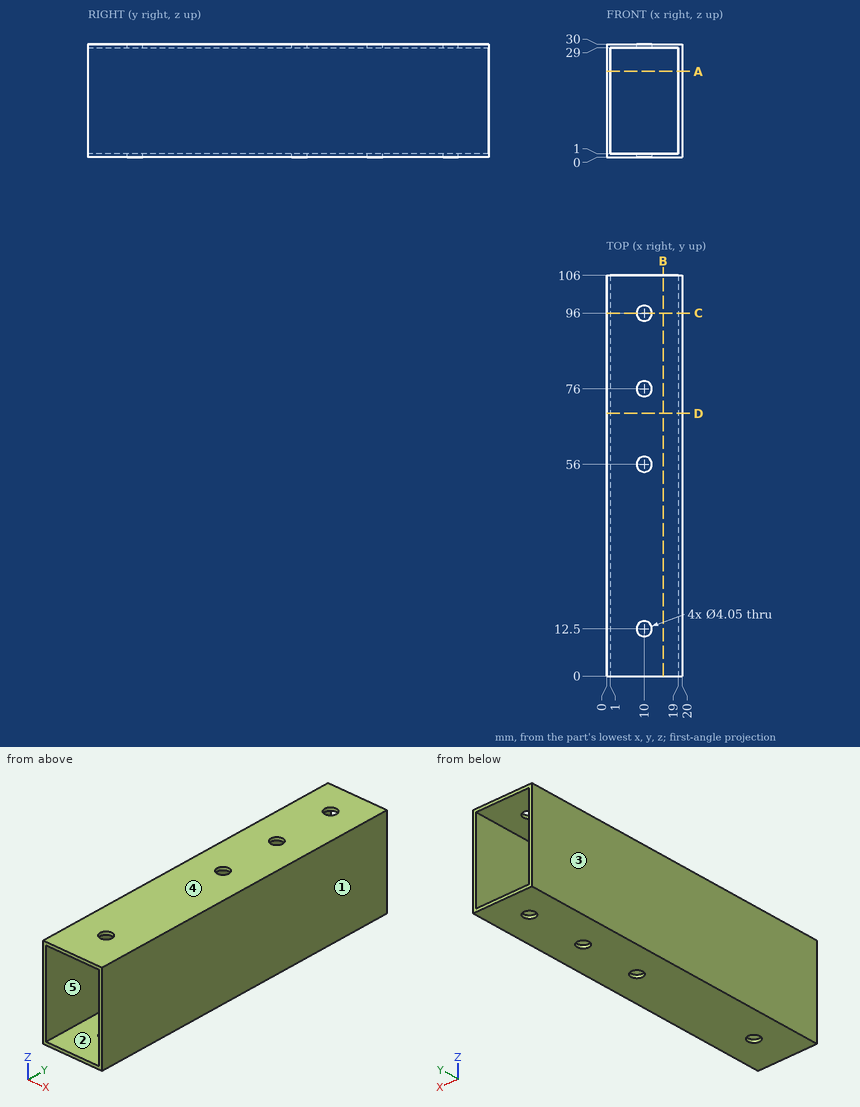
Part print with two shaded views. Sizes in mm from the minimum x, y, z corner. A direction names the side the tool comes from. Give positions to 0.01 mm unless a question says otherwise; leave off trailing zeros. Loops run counter-clockwise (first coordinate to the right, second up) from the corner with the lowest first, then second, coordinate; pieces in that order, holes last. Notation, with made-up numbers: (15, 54.5) - (29, 54.5) arc R26 ccw to (29, 74.5) - close; hole circle Ø9 at (1.5, -17.5). An arc over 180 degrees is marked (long way). Put each result on its own line as item: value.
Q1. Slice it at C-C (y = 96). Give the cut face in (x, z) (3 decimals), plus the area to 3 significant figures.
Filled in:
outline: (0, 0) - (7.975, 0) - (7.975, 1) - (1, 1) - (1, 29) - (7.975, 29) - (7.975, 30) - (0, 30) - close; (12.025, 0) - (20, 0) - (20, 30) - (12.025, 30) - (12.025, 29) - (19, 29) - (19, 1) - (12.025, 1) - close
area: 87.9 mm²
Q2. Mould opens along Z. For the marked faces 3, 4 and 5 say: pulls with the +Z half, pulls with the -Z half, needs draft (parallel to the pull), parting line crosses it, or undercut.
Filled in:
face 3: needs draft
face 4: pulls with the +Z half
face 5: undercut
Q3. Flat gauge pin, fed straight in: pin 1 (3 mm diameter, centred on x = 10, y = 12.5, fed in from +Z). Where does the tip first touch, or does it go through?
Filled in:
pin 1: passes through
Q4. Tool access for the marked faces 1 and 2: list every direction of +Z, -Z, +X, -X, +Y, -Y with a clear straight run to the whole face (end or side of a thin tool).
Filled in:
face 1: +Z, -Z, +X, +Y, -Y
face 2: +Y, -Y
Q5. Slice it at D-D (y = 69.5). Give the cut face in (x, z).
Filled in:
outline: (0, 0) - (20, 0) - (20, 30) - (0, 30) - close; hole (1, 1) - (19, 1) - (19, 29) - (1, 29) - close
Q6. Slice it at A-A (z = 22.75). Give the cut face in (x, y), plus the area to 3 significant figures.
Filled in:
outline: (0, 0) - (1, 0) - (1, 106) - (0, 106) - close; (19, 0) - (20, 0) - (20, 106) - (19, 106) - close
area: 212 mm²
Q7. Probe line 1 along Y through (x, z) = (10, 0.5) (3 decimals); line 2 along Z through (x, y) = (8.5, 26); line 3 along X through (y, z) = (63.5, 10). List the from-to ranges inside material, lowest first.
Filled in:
line 1: y = 0 to 10.475, 14.525 to 53.975, 58.025 to 73.975, 78.025 to 93.975, 98.025 to 106
line 2: z = 0 to 1, 29 to 30
line 3: x = 0 to 1, 19 to 20
Q8. Slice it at B-B (x = 15). Give the cut face in (y, z), plus the area to 3 significant figures.
Filled in:
outline: (0, 0) - (106, 0) - (106, 1) - (0, 1) - close; (0, 29) - (106, 29) - (106, 30) - (0, 30) - close
area: 212 mm²
